Job drawing, mm, ordinate dimensions from the low corner. One solid piece. A direction names the side the tool comes from. Round coordinates to 2 decimals unless told otherwise and drop trailing zeros. Order: outer loops, then holes, each group sorted by start corner. A loop starts at its lowest first (then second) coordinate and runs counter-clockwise, first axis right, second up. Notation, with made-up numbers: (70.5, 31) -> (91.5, 31) arc R5 ccw to (91.5, 38) -> close; hole circle Ø10 at (9.5, 44). An arc over 180 degrees is marked (long way). Answer as a JSON object with one key per item and string values. Group by question number.
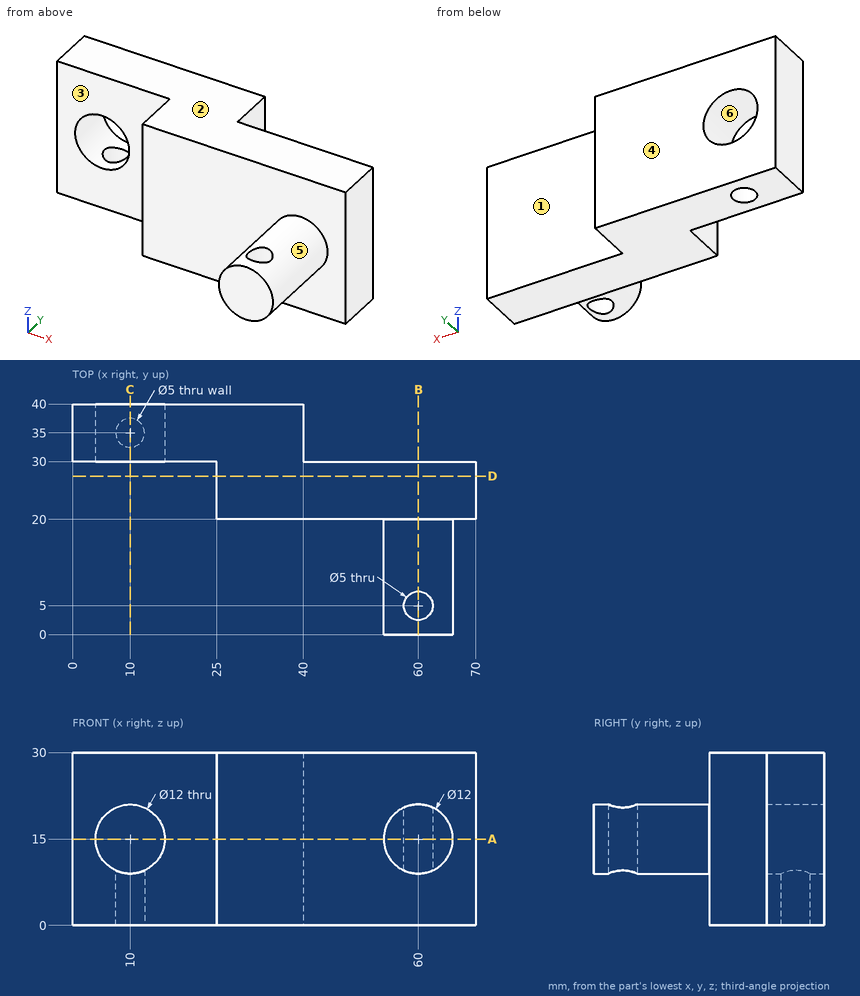
Q1. Band-saw the part on A-A (z = 15). List the corners of the cut face in (x, y), plus the area to 3 significant figures.
Q2. Band-saw the part on B-B (x = 60). List the corners of the cut face in (y, z).
Q3. Drop flat-ended pins along their axis: pin 1 Ø4 at (y, z) = (20.5, 21.5) entering from -X; pin 2 Ø4 at (y, z) = (7.5, 13) entering from -X; pin 3 Ø6 at (x, y) = (10, 35) entering from -Z; pin 4 Ø6 at (x, z) = (21, 8) entering from -Y. Give the stop position or say it passes through.
Q4. Which spindle directions (+Z, -Z, +X, -X, +Y, -Y) get a long thin tool onto all of the face, cutting with end or side? Do the marked faces 1, 2 and 3. Say none if no direction does.
Q5. Two-plate mould, pull along Z, no slides. Class the marked faces 4, 5 and 6: +Z half, -Z half, draft (parallel to the pull), parting line (faces both ways), or undercut.
Q6. Band-saw the part on C-C (x = 10). List the corners of the cut face in (y, z), plus the area to 3 significant figures.
Q7. Wall check: line 1 (Y direction, x = 10, z = 6); line 2 (Y direction, x = 60, z = 16); line 3 (Y direction, x = 33, z = 8.5). Give the ranges that are in metal, low to high. Write a range as [from, to].
Q8. Band-saw the part on D-D (y = 27.5). List the corners of the cut face in (x, z).
Completed:
{
 "1": {"outline": "(0, 30) -> (4, 30) -> (4, 40) -> (0, 40) -> close; (16, 30) -> (25, 30) -> (25, 20) -> (54, 20) -> (54, 0) -> (66, 0) -> (66, 20) -> (70, 20) -> (70, 30) -> (40, 30) -> (40, 40) -> (16, 40) -> close; hole circle Ø5 at (60, 5)", "area": "950 mm2"},
 "2": {"outline": "(0, 9) -> (2.5, 9) -> (2.5, 21) -> (0, 21) -> close; (7.5, 9) -> (20, 9) -> (20, 0) -> (30, 0) -> (30, 30) -> (20, 30) -> (20, 21) -> (7.5, 21) -> close"},
 "3": {"pin 1": "x = 25", "pin 2": "x = 54", "pin 3": "z = 0", "pin 4": "y = 30"},
 "4": {"face 1": "+Z, -Z, +X, +Y", "face 2": "+Z, +X, -X, +Y, -Y", "face 3": "+Z, -Z, -X, -Y"},
 "5": {"face 4": "draft", "face 5": "parting line", "face 6": "undercut"},
 "6": {"outline": "(30, 0) -> (32.5, 0) -> (32.5, 9) -> (30, 9) -> close; (30, 21) -> (40, 21) -> (40, 30) -> (30, 30) -> close; (37.5, 0) -> (40, 0) -> (40, 9) -> (37.5, 9) -> close", "area": "135 mm2"},
 "7": {"line 1": "[30, 32.5], [37.5, 40]", "line 2": "[0, 2.5], [7.5, 30]", "line 3": "[20, 40]"},
 "8": {"outline": "(25, 0) -> (70, 0) -> (70, 30) -> (25, 30) -> close"}
}
